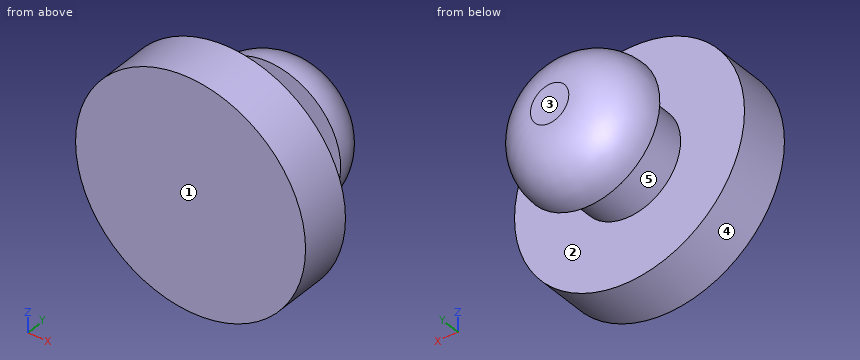
from build123d import *

# Parameters (mm, degrees)
SKETCH1_R           = 7.14375
BOSS_EXTRUDE1_DEPTH = 3.175
SKETCH2_R           = 3.175
BOSS_EXTRUDE2_DEPTH = 3.175
SKETCH3_R           = 4.365625
BOSS_EXTRUDE3_DEPTH = 3.175
FILLET1_R           = 3.175


with BuildPart() as part:
    # Sketch1 → Boss-Extrude1 (new body)
    with BuildSketch(Plane(origin=(0, 0, 0), x_dir=(1, 0, 0), z_dir=(0, 1, 0))):
        with Locations(Location((0, 0, 0), (0, 0, 270))):
            Circle(SKETCH1_R)
    extrude(amount=BOSS_EXTRUDE1_DEPTH)

    # Sketch2 → Boss-Extrude2 (add)
    with BuildSketch(Plane(origin=(0, 3.175, 0), x_dir=(1, 0, 0), z_dir=(0, 1, 0))):
        with Locations(Location((0, 0, 0), (0, 0, 270))):
            Circle(SKETCH2_R)
    extrude(amount=BOSS_EXTRUDE2_DEPTH)

    # Sketch3 → Boss-Extrude3 (add)
    with BuildSketch(Plane(origin=(0, 6.35, 0), x_dir=(1, 0, 0), z_dir=(0, 1, 0))):
        with Locations(Location((0, 0, 0), (0, 0, 270))):
            Circle(SKETCH3_R)
    extrude(amount=BOSS_EXTRUDE3_DEPTH)

    # Fillet1
    fillet1_edges = [part.edges().sort_by_distance(p)[0] for p in [
        (0, 9.525, -4.365625),
    ]]
    fillet(fillet1_edges, radius=FILLET1_R - 0.0001)  # a hair under: the kernel refuses the full size


solid = part.part
For this review, take the finished solid that the model builds, in its own axes (mm). Face numbers are marked on the shaded views. A direction names the side the tool comes from. Give positions to 0.01 mm unless a question says otherwise; leave off trailing zeros. Loops run counter-clockwise (first coordinate to the right, second up) from the corner with the lowest first, then second, coordinate; pieces in that order, holes last. Notation, with made-up numbers: M 28,46.25 L 33,46.25 A15 cw 33,51.25 Z; hole C 12,16 d1. An arc over 180 degrees is marked long. Answer as a JSON object with one key per item and string values. Group by question number.
Q1. Add section A-A on x = 6.5. Give the boundary of the cut face in (y, z) (3 decimals).
Q2. Insertion check: P1, Ø1, axis at y = 8, z = -3.5, coming from the +X side; P2, Ø2, axis at x = 5, y = 3.5, coming from the +Z side; P3, Ø1.5, axis at y = 8.5, z = 1.5, coming from the +X side. Each pin has a flat end and moves straight along its axis. Give the tip position at first contact, or say it passes through.
Q3. Mouldability with a two-part tool opening along Y and no side actions: class the marked faces 1, 2 and 3 as +Y half, -Y half, draft (parallel to the pull), parting line (faces both ways), or undercut.
Q4. For probe 1 along Y at (x, z) = (-4, -5) (3 decimals); probe 2 along Y at (x, z) = (1.75, -3) (3 decimals); probe 3 along X at (y, z) = (3.75, -2.25), list the stretches that pass through material, from the lowest coordinate up. Write a range as [from, to].
Q5. Tool access review of the marked faces 4 and 5: name each direction out of +Z, -Z, +X, -X, +Y, -Y from which nothing blocks a thin tool from reaching the whole face with its end or side.
Q6. Add section B-B on z = -5.75. Give the boundary of the cut face in (x, y) (3 decimals).
Checked values:
{
 "1": {"outline": "M 0,-2.964 L 3.175,-2.964 L 3.175,2.964 L 0,2.964 Z"},
 "2": {"P1": "x = 2.63", "P2": "z = 5.88", "P3": "x = 3.83"},
 "3": {"face 1": "-Y half", "face 2": "undercut", "face 3": "+Y half"},
 "4": {"probe 1": "[0, 3.175]", "probe 2": "[0, 3.175], [6.35, 8.557]", "probe 3": "[-2.24, 2.24]"},
 "5": {"face 4": "+Y, -Y", "face 5": "none"},
 "6": {"outline": "M -4.239,0 L 4.239,0 L 4.239,3.175 L -4.239,3.175 Z"}
}
